The model under review builds one solid part; all positions refer to its coordinate system, in mm. A direction names the side the tool comes from. Coordinates: 2 decimals unless noted, no trailing zeros. Loops run counter-clockwise (first coordinate to the right, second up) from the corner with the lowest first, then second, coordinate; pieces in that order, holes last. Notation, with made-up numbers: (49, 52.5) -> (95, 52.5) arc R21 cw to (95, 56.5) -> close; hole circle Ø6 at (87.25, -0.5). An arc over 180 degrees is marked (long way). One line per question, with ' | ' between items. Start each with the question number.
from build123d import *

# Parameters (mm, degrees)
SKETCH1_W                                         = 101.6
SKETCH1_H                                         = 23.0124
BOSS_EXTRUDE1_DEPTH                               = 4.7625
CBORE_FOR_5_16_SOCKET_HEAD_CAP_SCREW1_D           = 8.2042
CBORE_FOR_5_16_SOCKET_HEAD_CAP_SCREW1_CBORE_D     = 13.49502
CBORE_FOR_5_16_SOCKET_HEAD_CAP_SCREW1_CBORE_DEPTH = 1.5875
CBORE_FOR_6_SOCKET_HEAD_CAP_SCREW1_D              = 3.6576
CBORE_FOR_6_SOCKET_HEAD_CAP_SCREW1_CBORE_D        = 7.14502
CBORE_FOR_6_SOCKET_HEAD_CAP_SCREW1_CBORE_DEPTH    = 3.5052
FILLET1_R                                         = 2.54


with BuildPart() as part:
    # Sketch1 → Boss-Extrude1 (new body)
    with BuildSketch(Plane.XY):
        with Locations((50.8, 11.5062)):
            Rectangle(SKETCH1_W, SKETCH1_H)
    extrude(amount=BOSS_EXTRUDE1_DEPTH)

    # CBORE for 5/16 Socket Head Cap Screw1 (through all)
    with Locations(Plane.XY.offset(4.7625)):
        with Locations((76.2, 9.525), (25.4, 9.525)):
            CounterBoreHole(CBORE_FOR_5_16_SOCKET_HEAD_CAP_SCREW1_D / 2, CBORE_FOR_5_16_SOCKET_HEAD_CAP_SCREW1_CBORE_D / 2, CBORE_FOR_5_16_SOCKET_HEAD_CAP_SCREW1_CBORE_DEPTH)

    # CBORE for #6 Socket Head Cap Screw1 (through all)
    with Locations(Plane(origin=(0, 0, 0), x_dir=(-1, 0, 0), z_dir=(0, 0, -1))):
        with Locations((-55.218690757, 15.7734), (-55.218690757, 4.8514)):
            CounterBoreHole(CBORE_FOR_6_SOCKET_HEAD_CAP_SCREW1_D / 2, CBORE_FOR_6_SOCKET_HEAD_CAP_SCREW1_CBORE_D / 2, CBORE_FOR_6_SOCKET_HEAD_CAP_SCREW1_CBORE_DEPTH)

    # Fillet1
    fillet1_edges = [part.edges().sort_by_distance(p)[0] for p in [
        (101.6, 0, 2.38125),
        (0, 0, 2.38125),
    ]]
    fillet(fillet1_edges, radius=FILLET1_R)


solid = part.part
1) Consider section B-B, the plane y = 11. Write out the cut boundary in (x, z) (1 decimal), plus the area to 3 significant figures.
2) Consider section C-C, the plane z = 1.75. Write out the cut boundary in (x, y) (1 decimal), plus the area to 3 significant figures.
3) Insertion check: pin 1 Ø9.5 at (x, y) = (55.22, 15.77) entering from -Z; pin 2 Ø3.5 at (x, y) = (54.5, 4.5) entering from -Z; pin 3 Ø6.5 at (x, y) = (25.4, 9.525) entering from -Z. Each pin has a flat end and moves straight along its axis. Give the tip position at first contact, or say it passes through.
4) Mouldability with a two-part tool opening along Y and no side actions: class faces 4 (the face through (50, 12, 4.762)), 5 (the face through (29.027, 15.215, 3.98)), 6 (the face through (50, 23.012, 2)) as +Y half, -Y half, draft (parallel to the pull), parting line (faces both ways), or undercut.
5) Wall thickness on L1, parallel to X at y = 12.25, z = 4.6; L2, parallel to X at y = 10.75, z = 3.95; L3, parallel to Y at x = 54.5, z = 1.05: over which ranges is each line inside the solid? List them lowest first.
6) Consider section A-A, the plane x = 76.2. Write out the cut boundary in (y, z) (1 decimal), plus the area to 3 significant figures.
7) Machinability: for faces 1 (the face through (69.46, 9.82, 3.98)), 2 (the face through (57, 17, 3.505)), 3 (the face through (72.3, 10.8, 1.6)), which of the approach directions +Z, -Z, +X, -X, +Y, -Y give a long, thin tool a straight path to every point of the face, cutting with its end or side? Answer none if there is none.
Filled sheet:
1) outline: (0, 0) -> (21.6, 0) -> (21.6, 3.2) -> (18.8, 3.2) -> (18.8, 4.8) -> (0, 4.8) -> close; (29.2, 0) -> (72.4, 0) -> (72.4, 3.2) -> (69.6, 3.2) -> (69.6, 4.8) -> (32, 4.8) -> (32, 3.2) -> (29.2, 3.2) -> close; (80, 0) -> (101.6, 0) -> (101.6, 4.8) -> (82.8, 4.8) -> (82.8, 3.2) -> (80, 3.2) -> close | area: 393 mm^2
2) outline: (0, 2.5) arc R2.5 ccw to (2.5, 0) -> (99.1, 0) arc R2.5 ccw to (101.6, 2.5) -> (101.6, 23) -> (0, 23) -> close; hole circle Ø8.2 at (25.4, 9.5); hole circle Ø7.1 at (55.2, 4.9); hole circle Ø7.1 at (55.2, 15.8); hole circle Ø8.2 at (76.2, 9.5) | area: 2,150 mm^2
3) pin 1: z = 0 | pin 2: z = 3.51 | pin 3: through
4) face 4: draft | face 5: undercut | face 6: +Y half
5) L1: 0 to 19.23, 31.57 to 70.03, 82.37 to 101.6 | L2: 0 to 18.76, 32.04 to 69.56, 82.84 to 101.6 | L3: 0 to 1.35, 8.35 to 12.27, 19.27 to 23.01
6) outline: (0, 0) -> (5.4, 0) -> (5.4, 3.2) -> (2.8, 3.2) -> (2.8, 4.8) -> (0, 4.8) -> close; (13.6, 0) -> (23, 0) -> (23, 4.8) -> (16.3, 4.8) -> (16.3, 3.2) -> (13.6, 3.2) -> close | area: 62.1 mm^2
7) face 1: +Z | face 2: -Z | face 3: +Z, -Z
